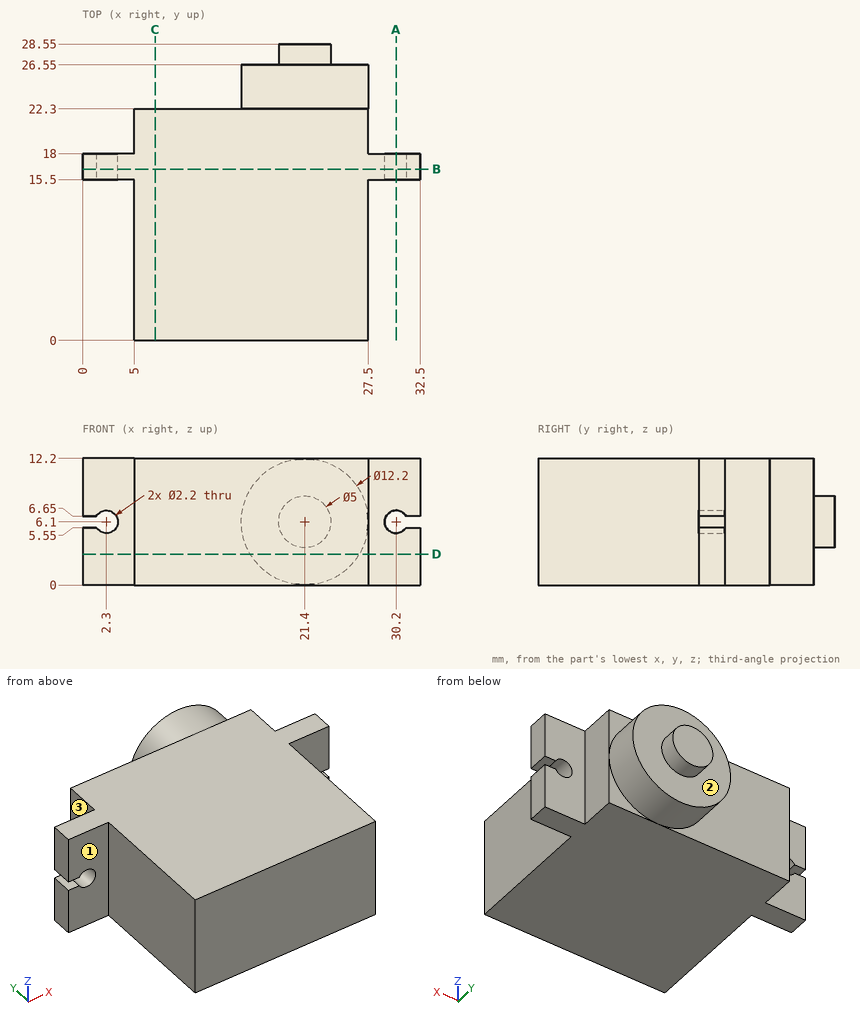
Print and shaded views of the part. All mm, measured from the part's lowest x, y and z. A direction names the side the tool comes from. Round coordinates to 2 decimals unless told otherwise and drop trailing zeros. Loops run counter-clockwise (first coordinate to the right, second up) from the corner with the lowest first, then second, coordinate; pieces in that order, holes last. Notation, with made-up numbers: (68, 77) -> (86, 77) arc R17 ccw to (86, 84) -> close; hole circle Ø2 at (15.5, -12.75). An arc over 180 degrees is marked (long way). Use CSV: the item, a comma, the result in double quotes. Start each with the question number.
1) Which spindle directions (+Z, -Z, +X, -X, +Y, -Y) get a long thin tool onto all of the face, cutting with end or side? Do the marked faces 1, 2 and 3. Say none if no direction does.
2) Cut at A-A, the plane x = 30.2. Write the cut outline in (y, z), plus the area to 3 significant figures.
3) Wall check: L1, parallel to Z at x = 30.2, y = 17.35; L2, parallel to Y at x = 25, z = 6; L3, parallel to X at y = 16.8, z = 6.1. Give the ranges that are in metal, low to high. Write a range as [from, to].
4) Cut at D-D, the plane z = 3. Write the cut outline in (x, y), plus the area to 3 significant figures.
5) Cut at B-B, the plane y = 16.5. Write the cut outline in (x, z).
6) Drop flat-ended pins along their axis: P1, Ø3, axis at x = 30.2, z = 6.1, coming from the -Y side; P2, Ø4, axis at x = 15, z = 1.5, coming from the +Y side; P3, Ø1.5, axis at x = 2, z = 5, coming from the +Y side. Give the stop position or say it passes through.
7) Cut at C-C, the plane x = 7. Write the cut outline in (y, z), plus the area to 3 significant figures.
Determined:
1,face 1,"+Z, -Z, -X, -Y"
1,face 2,"+Y"
1,face 3,"+Z, -Z, -X, +Y"
2,outline,"(15.5, 0) -> (18, 0) -> (18, 5) -> (15.5, 5) -> close; (15.5, 7.2) -> (18, 7.2) -> (18, 12.2) -> (15.5, 12.2) -> close"
2,area,"25.0 mm2"
3,L1,"z = [0, 5], [7.2, 12.2]"
3,L2,"y = [0, 26.55]"
3,L3,"x = [3.4, 29.1]"
4,outline,"(0, 15.5) -> (5, 15.5) -> (5, 0) -> (27.5, 0) -> (27.5, 15.5) -> (32.5, 15.5) -> (32.5, 18) -> (27.5, 18) -> (27.5, 22.3) -> (26.65, 22.3) -> (26.65, 26.55) -> (16.15, 26.55) -> (16.15, 22.3) -> (5, 22.3) -> (5, 18) -> (0, 18) -> close"
4,area,"571 mm2"
5,outline,"(0, 0) -> (32.5, 0) -> (32.5, 5.55) -> (31.15, 5.55) arc R1.1 cw (long way) to (31.15, 6.65) -> (32.5, 6.65) -> (32.5, 12.2) -> (0, 12.2) -> (0, 6.65) -> (1.35, 6.65) arc R1.1 cw (long way) to (1.35, 5.55) -> (0, 5.55) -> close"
6,P1,"stops at y = 15.5"
6,P2,"stops at y = 26.55"
6,P3,"stops at y = 18"
7,outline,"(0, 0) -> (22.3, 0) -> (22.3, 12.2) -> (0, 12.2) -> close"
7,area,"272 mm2"
